Part model, mm, in its own coordinate system. Round coordinates to 2 decimals unless told otherwise and drop trailing zeros. Order: outer loops, then holes, each group sorted by start corner. A loop starts at its lowest first (then second) coordinate and runs counter-clockwise, first axis right, second up. Notation, with made-up numbers: (-11, -23) - (33, -23) arc R30 cw to (33, -1) - close; hole circle Ø10 at (65, 80). An arc over 180 degrees is marked (long way). Return JSON: item names as keys, results as strings. Group by question number.
Item 1: Saw through at A-A on z = 2.25. State how many separate pieces and enclosed holes the cut face has, and give its area (3 significant figures).
Item 2: Probe probe 1 along X at (y, z) = (12.5, 1.25); probe 2 along X at (y, z) = (-10.5, 8.5); probe 3 along Y at (x, z) = (-98, 2.5). List the from-to ranges inside material, lowest first.
Item 3: Two-plate mould, pull along X, no slides. Class faces 1 (the face through (27, 2, 10)), 2 (the face through (-2.17, -9.76, 5.07)), 3 (the face through (123.997, 39.048, 4.93)): released by +X, released by -X, zero draft, split by the parting line, or undercut.
Item 4: Drop flat-ended pins along their axis: pin 1 (5 mm diameter, centred on x = 83.5, z = 5.5, fed in from -Y); pin 2 (4 mm diameter, centred on y = 8, z = 2, fed in from +X); pin 3 (4 mm diameter, centred on x = 57.5, y = -99.59, fed in from -Z); pin 4 (1 mm diameter, centred on x = -68, z = 3.5, fed in from +Y). Give the stop position or say it passes through.
Item 5: Saw through at B-B on x = 91. List the corners of the cut face in (y, z), and give its area (3 significant figures).
```python
from build123d import *

# Parameters (mm, degrees)
SKETCH_1_R          = 130
EXTRUDE_1_DEPTH     = 10
SKETCH_7_R          = 2.5
CUT_EXTRUDE_3_DEPTH = 10
SKETCH_9_R          = 10
CUT_EXTRUDE_5_DEPTH = 185.119526395
SKETCH_10_R         = 2.5
CUT_EXTRUDE_6_DEPTH = 185.119526395


with BuildPart() as part:
    # 草图1 → 凸台-拉伸1 (new body)
    with BuildSketch(Plane.XY):
        Circle(SKETCH_1_R)
    extrude(amount=EXTRUDE_1_DEPTH)

    # 草图7 → 切除-拉伸3 (cut)
    with BuildSketch(Plane(origin=(0, 0, 0), x_dir=(-1, 0, 0), z_dir=(0, 0, -1))):
        with Locations((0, 70)):
            Circle(SKETCH_7_R)
        with Locations((60.621778265, 35)):
            Circle(SKETCH_7_R)
        with Locations((60.621778265, -35)):
            Circle(SKETCH_7_R)
        with Locations((0, -70)):
            Circle(SKETCH_7_R)
        with Locations((-60.621778265, -35)):
            Circle(SKETCH_7_R)
        with Locations((-60.621778265, 35)):
            Circle(SKETCH_7_R)
        with Locations((57.5, 99.592921435)):
            Circle(SKETCH_7_R)
        with Locations((99.592921435, 57.5)):
            Circle(SKETCH_7_R)
        with Locations((115, 0)):
            Circle(SKETCH_7_R)
        with Locations((99.592921435, -57.5)):
            Circle(SKETCH_7_R)
        with Locations((57.5, -99.592921435)):
            Circle(SKETCH_7_R)
        with Locations((0, -115)):
            Circle(SKETCH_7_R)
        with Locations((-57.5, -99.592921435)):
            Circle(SKETCH_7_R)
        with Locations((-99.592921435, -57.5)):
            Circle(SKETCH_7_R)
        with Locations((-115, 0)):
            Circle(SKETCH_7_R)
        with Locations((-99.592921435, 57.5)):
            Circle(SKETCH_7_R)
        with Locations((-57.5, 99.592921435)):
            Circle(SKETCH_7_R)
        with Locations((0, 115)):
            Circle(SKETCH_7_R)
    extrude(amount=-CUT_EXTRUDE_3_DEPTH, mode=Mode.SUBTRACT)

    # 草图9 → 切除-拉伸5 (cut, through all)
    with BuildSketch(Plane.XY.offset(10)):
        Circle(SKETCH_9_R)
    extrude(amount=-CUT_EXTRUDE_5_DEPTH, mode=Mode.SUBTRACT)

    # 草图10 → 切除-拉伸6 (cut, through all)
    with BuildSketch(Plane.XY.offset(10)):
        with Locations((0, 22.5)):
            Circle(SKETCH_10_R)
        with Locations((19.485571585, 11.25)):
            Circle(SKETCH_10_R)
        with Locations((19.485571585, -11.25)):
            Circle(SKETCH_10_R)
        with Locations((0, -22.5)):
            Circle(SKETCH_10_R)
        with Locations((-19.485571585, -11.25)):
            Circle(SKETCH_10_R)
        with Locations((-19.485571585, 11.25)):
            Circle(SKETCH_10_R)
    extrude(amount=-CUT_EXTRUDE_6_DEPTH, mode=Mode.SUBTRACT)


solid = part.part
```
Filled in:
{
 "1": {"separate pieces": "1", "enclosed holes": "25", "area": "52,300 mm^2"},
 "2": {"probe 1": "x = -129.4 to -21.65, -17.32 to 17.32, 21.65 to 129.4", "probe 2": "x = -129.58 to -21.87, -17.1 to 17.1, 21.87 to 129.58", "probe 3": "y = -85.42 to -59.43, -55.57 to 55.57, 59.43 to 85.42"},
 "3": {"face 1": "zero draft", "face 2": "undercut", "face 3": "split by the parting line"},
 "4": {"pin 1": "stops at y = -101.68", "pin 2": "stops at x = 129.86", "pin 3": "passes through", "pin 4": "stops at y = 111.1"},
 "5": {"outline": "(-92.84, 0) - (92.84, 0) - (92.84, 10) - (-92.84, 10) - close", "area": "1,860 mm^2"}
}
